Source: CAD feature listing. Evaluate the final solid. Frame: model axes, mm. A direction names the side the tool comes from. Give positions to 0.01 mm unless a question says otherwise; leave off trailing zeros. Order: outer loops, then holes, each group sorted by start corner. A loop starts at its lowest first (then second) coordinate and runs counter-clockwise, first axis right, second up.
Autodesk Inventor part; units mm, degrees
ref_plane "YZ Plane" through (0, 0, 0) normal (1, 0, 0) x (0, 1, 0)
ref_plane "XZ Plane" through (0, 0, 0) normal (0, 1, 0) x (-1, 0, 0)
ref_plane "XY Plane" through (0, 0, 0) normal (0, 0, 1) x (1, 0, 0)
sketch "Sketch1" plane through (0, 0, 0) normal (0, 1, 0) x (-1, 0, 0)
  line L0 (20, -15) -> (-20, -15)
  line L1 (-20, -15) -> (-20, 15)
  line L2 (-20, 15) -> (20, 15)
  line L3 (20, 15) -> (20, -15)
  line L4 (20, -15) -> (-20, 15) construction
  line L5 (-20, -15) -> (20, 15) construction
  point P0 (0, 0)
  dimension "d0" = 40
  dimension "d1" = 30
extrude "Plate1" add sketch "Sketch1" along normal blind 1.5
sketch "Sketch2" plane through (18.5, 1.5, 15) normal (1, 0, 0) x (0, 1, 0)
  line L0 (0, -30) -> (0, 0)
  line L1 (0, 0) -> (-22, 0)
  line L2 (-22, 0) -> (-22, -30)
  line L3 (-22, -30) -> (0, -30)
edge flange "Flange1" height 22 angle 90 thickness 1.5 bend radius 0.31 thickness toward (1, 0, 0) relief tear relief width 1.5 relief depth 0.75 corner gap 0.31 corner form 0 edges at (20, 0, 0) (-20, 0, 0) wall of the first edge with corners at (18.5, 1.5, -15) (18.5, 1.5, 15) (18.5, -20.5, 15) (18.5, -20.5, -15)
bend "Bend1"
corner "Corner1"
sketch "Sketch3" plane through (20, -20.5, 15) normal (1, 0, 0) x (0, 0, -1)
  circle A0 centre (20, 5.19) radius 1.55
  circle A1 centre (10, 5.19) radius 1.55
  line L0 (30, 20.19) -> (0, 20.19)
  line L1 (30, 0) -> (30, 20.19)
  point P0 (15, 20.5)
  dimension "d13" = 3.1
  dimension "d14" = 3.1
  dimension "d15" = 15
  dimension "d16" = 15
  dimension "d17" = 10
  dimension "d33" = 10
extrude "Cut1" cut sketch "Sketch3" against normal through all
sketch "Sketch4" plane through (0, 1.5, 0) normal (0, 1, 0) x (1, 0, 0)
  circle A0 centre (8, -7) radius 4
  circle A1 centre (-8, -7) radius 4
  arc A2 (0, 10) -> (-8.6603, 5) centre (0, 0) ccw construction
  arc A3 (0, 12.5) -> (-10.8253, 6.25) centre (0, 0) ccw
  arc A4 (0, 7.5) -> (-6.4952, 3.75) centre (0, 0) ccw
  arc A5 (0, 7.5) -> (0, 12.5) centre (0, 10) ccw
  arc A6 (-10.8253, 6.25) -> (-6.4952, 3.75) centre (-8.6603, 5) ccw
  line L0 (0, 0) -> (-8.6603, 5) construction
  line L1 (0, 0) -> (0, 10) construction
  arc A7 (8.6603, 5) -> (0, 10) centre (0, 0) ccw construction
  arc A8 (10.8253, 6.25) -> (0, 12.5) centre (0, 0) ccw
  arc A9 (6.4952, 3.75) -> (0, 7.5) centre (0, 0) ccw
  arc A10 (6.4952, 3.75) -> (10.8253, 6.25) centre (8.6603, 5) ccw
  arc A11 (0, 12.5) -> (0, 7.5) centre (0, 10) ccw
  line L2 (0, 0) -> (8.6603, 5) construction
  line L3 (0, 0) -> (0, 10) construction
  dimension "d20" = 8
  dimension "d21" = 8
  dimension "d22" = 10
  dimension "d23" = 60
  dimension "d24" = 5
  dimension "d25" = 60
  dimension "d26" = 5
  dimension "d27" = 7
  dimension "d28" = 7
  dimension "d29" = 8
  dimension "d30" = 8
extrude "Cut2" cut sketch "Sketch4" against normal through all
equation "\"d16\" = d15"
equation "\"d18\" = Thickness"
equation "\"d31\" = Thickness"
equation "\"d2\" = Thickness"
equation "\"d3\" = BendReliefWidth"
equation "\"d4\" = BendReliefDepth"
equation "\"d5\" = MinimumRemnant"
equation "\"d6\" = TransitionRadius"
equation "\"d9\" = BendRadius"
equation "\"d10\" = CornerReliefSize"
equation "\"d11\" = GapSize"
equation "\"d12\" = JacobiRadiusSize"
equation "\"BendReliefWidth\" = Thickness"
equation "\"BendReliefDepth\" = 0.5 * Thickness"
equation "\"CornerReliefSize\" = 4 * Thickness"
equation "\"MinimumRemnant\" = 2 * Thickness"
equation "\"TransitionRadius\" = BendRadius"
equation "\"JacobiRadiusSize\" = BendRadius"
equation "\"GapSize\" = Thickness"
properties part number "Head2" material "Aluminum 6061-AHC"
1) Section query A-A on y = -7. Output: boundary loops of the cut face in (x, z).
Checks:
outline: (-20, -15) - (-18.5, -15) - (-18.5, 15) - (-20, 15) - close; (18.5, -15) - (20, -15) - (20, 15) - (18.5, 15) - close
2) Ray query, L1, parallel to X at y = -9, z = 5.5; L2, parallel to X at y = 0.8, z = 7; L3, parallel to Z at x = -8, y = 0.8. Return the intervals inside material, ascending.
Checks:
L1: x = -20 to -18.5, 18.5 to 20
L2: x = -19.62 to -12, -4 to 4, 12 to 19.62
L3: z = -15 to -9.6, -2.59 to 3, 11 to 15
3) Pull-direction query (X, two-part tool) for faces 1 (the face through (20, -11, 0)), 2 (the face through (-19, -20.5, 0)), 3 (the face through (4.8, 0.8, 9.4)); classes: +X half, -X half, draft (parallel to the pull), parting line (faces both ways), or undercut.
Checks:
face 1: +X half
face 2: draft
face 3: undercut
4) First-contact query: pin 1 Ø15 at (x, z) = (6, -4.5) entering from -Y; pin 2 Ø3 at (y, z) = (-15.31, -5) entering from +X. Flat tips, straight axial feed; report the tip coordinate or a pass-through.
Checks:
pin 1: stops at y = 0
pin 2: passes through
5) Section query D-D on y = -15.31. Output: boundary loops of the cut face in (x, z).
Checks:
outline: (-20, -15) - (-18.5, -15) - (-18.5, -6.55) - (-20, -6.55) - close; (-20, -3.45) - (-18.5, -3.45) - (-18.5, 3.45) - (-20, 3.45) - close; (-20, 6.55) - (-18.5, 6.55) - (-18.5, 15) - (-20, 15) - close; (18.5, -15) - (20, -15) - (20, -6.55) - (18.5, -6.55) - close; (18.5, -3.45) - (20, -3.45) - (20, 3.45) - (18.5, 3.45) - close; (18.5, 6.55) - (20, 6.55) - (20, 15) - (18.5, 15) - close
6) Section query C-C on x = 8. Output: boundary loops of the cut face in (y, z), and give its area (3 significant figures).
Checks:
outline: (0, -15) - (1.5, -15) - (1.5, -9.6) - (0, -9.6) - close; (0, -2.59) - (1.5, -2.59) - (1.5, 3) - (0, 3) - close; (0, 11) - (1.5, 11) - (1.5, 15) - (0, 15) - close
area: 22.5 mm2
7) Reachability of faces 4 (the face through (-3.702, 0.76, -6.523)), 5 (the face through (0.1, 0.2, -15)), 6 (the face through (0, 0, 0)) from +Z, -Z, +X, -X, +Y, -Y: full face, straight path, thin tool, end or side. Return the list, or none.
Checks:
face 4: +Y, -Y
face 5: -Z, +X, -X, +Y, -Y
face 6: +Z, -Z, -Y
8) Section query B-B on z = 7. Output: boundary loops of the cut face in (x, y), and give its area (3 significant figures).
Checks:
outline: (-20, -20.5) - (-18.5, -20.5) - (-18.5, -0.31) arc R0.31 cw to (-18.19, 0) - (-12, 0) - (-12, 1.5) - (-18.19, 1.5) arc R1.81 ccw to (-20, -0.31) - close; (-4, 0) - (4, 0) - (4, 1.5) - (-4, 1.5) - close; (12, 0) - (18.19, 0) arc R0.31 cw to (18.5, -0.31) - (18.5, -20.5) - (20, -20.5) - (20, -0.31) arc R1.81 ccw to (18.19, 1.5) - (12, 1.5) - close
area: 96.1 mm2
